Input: part model. Units: mm. Frame: model coordinates. A direction names the side the tool comes from. Coordinates: 2 decimals unless noted, no trailing zeros. Order: outer loops, then holes, each group sorted by start corner. A loop starts at its lowest first (then second) coordinate and runs counter-clockwise, first axis right, second up. Notation, with made-up numbers: (-26, 5) -> (-15, 5) arc R21 ccw to (-15, 37) -> close; hole circle Ø7 at (81.5, 79). An arc over 180 degrees is marked (long way). Answer as CSV lines item,"result".
Autodesk Inventor part; units mm, degrees
ref_plane "YZ Plane" through (0, 0, 0) normal (1, 0, 0) x (0, 1, 0)
ref_plane "XZ Plane" through (0, 0, 0) normal (0, 1, 0) x (-1, 0, 0)
ref_plane "XY Plane" through (0, 0, 0) normal (0, 0, 1) x (1, 0, 0)
sketch "Sketch1" plane through (0, 0, 0) normal (0, 1, 0) x (-1, 0, 0)
  line L0 (-3.8257, 4.2576) -> (4.1137, 4.2576) construction
  line L1 (4.1137, 4.2576) -> (4.1137, -4.4222) construction
  line L2 (4.1137, -4.4222) -> (-3.8257, -4.4222) construction
  line L3 (-3.8257, -4.4222) -> (-3.8257, 4.2576) construction
  line L4 (12.4147, -21.2247) -> (0.0234, -21.2247)
  line L5 (0.0234, -21.2247) -> (0.0234, -18.6312)
  line L6 (0.0234, -18.6312) -> (4.6341, -18.6312)
  line L7 (4.6341, -18.6312) -> (4.6341, -1.6087)
  line L8 (4.6341, -1.6087) -> (0.0234, -1.6087)
  line L9 (0.0234, -1.6087) -> (0.0234, 0.7173)
  spline S0 degree 2 poles (0.0234, 0.7173) (2.6375, 0.7173) (5.1075, 2.1993) (5.2722, 4.2576) knots 0 0 0 1 2 2 2
  line L10 (5.2722, 4.2576) -> (7.9069, 4.2576)
  line L11 (7.9069, 4.2576) -> (7.9069, -18.6312)
  line L12 (7.9069, -18.6312) -> (12.4147, -18.6312)
  line L13 (12.4147, -18.6312) -> (12.4147, -21.2247)
  point P0 (0, 0)
extrude "Extrusion1" add sketch "Sketch1" along normal blind 12.7
properties part number "Text1"
1. Contact query for flat-ended pins moving along their axis: pin 1 (6.5 mm diameter, centred on y = 6, z = -10.5, fed in from -X); pin 2 (1.4 mm diameter, centred on x = -11, y = 6.5, fed in from +Z); pin 3 (1.4 mm diameter, centred on x = -3, y = 6.5, fed in from +Z). Output: stop coordinate, or through.
Findings:
pin 1,"stops at x = -7.91"
pin 2,"stops at z = -18.63"
pin 3,"stops at z = 1.36"
2. Cut plane A-A (z = -4.5). Return the cut outline in (x, y).
Findings:
outline,"(-7.91, 0) -> (-4.63, 0) -> (-4.63, 12.7) -> (-7.91, 12.7) -> close"
3. Cut plane B-B (x = -10). Return the cut outline in (y, z).
Findings:
outline,"(0, -21.22) -> (12.7, -21.22) -> (12.7, -18.63) -> (0, -18.63) -> close"
4. Reachability of faces 1 (the face through (-0.023, 6, -20)), 2 (the face through (-2, 6, -18.631)), 3 (the face through (-7.907, 6, -7)) from +Z, -Z, +X, -X, +Y, -Y: full face, straight path, thin tool, end or side. Return the list, or none.
Findings:
face 1,"+Z, -Z, +X, +Y, -Y"
face 2,"+X, +Y, -Y"
face 3,"+Z, -X, +Y, -Y"
5. Ray query, line 1 along X through (y, z) = (5.75, -3.75); line 2 along Z through (x, y) = (-10, 1); line 3 along Z through (x, y) = (-4.5, 11.5). Return the intervals inside material, ascending.
Findings:
line 1,"x = -7.91 to -4.63"
line 2,"z = -21.22 to -18.63"
line 3,"z = -21.22 to -18.63, -1.61 to 2"
